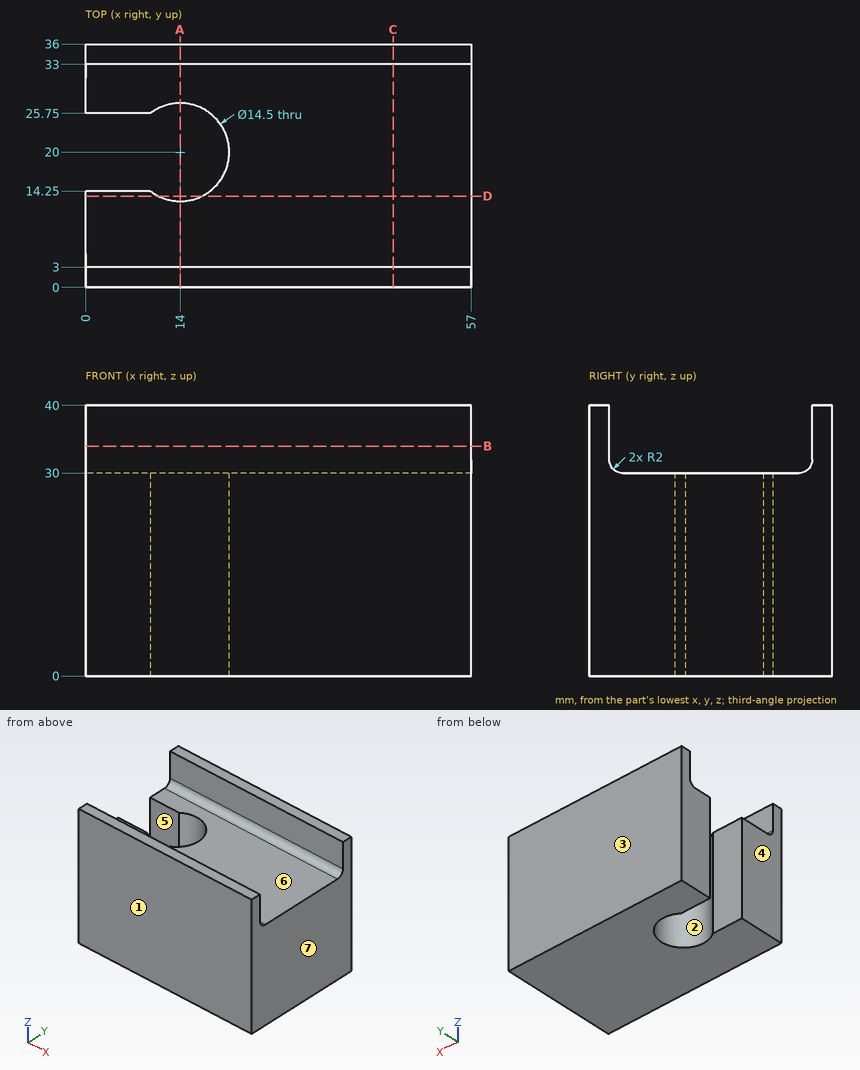
Verification items for this drawing (mm, ordinates from the low corner). A direction names the side the tool comes from. Round coordinates to 2 decimals unless told otherwise and drop trailing zeros. Order: outer loops, then holes, each group sorted by start corner. A loop starts at its lowest first (then second) coordinate and runs counter-clockwise, first axis right, second up.
1) Cross-section at D-D, the plane y = 13.5. Record the cut outline in (x, z), plus the area to 3 significant figures.
Geometry says:
outline: (0, 0) - (10.79, 0) - (10.79, 30) - (0, 30) - close; (17.21, 0) - (57, 0) - (57, 30) - (17.21, 30) - close
area: 1,520 mm2
2) Material ranges on line 1 (Y direction, x = 14, z = 22.75); line 2 (Y direction, x = 34, z = 38.5); line 3 (Z direction, x = 30, y = 16.5), recorded low to high.
Geometry says:
line 1: y = 0 to 12.75, 27.25 to 36
line 2: y = 0 to 3, 33 to 36
line 3: z = 0 to 30
3) Cross-section at B-B, the plane z = 34. Record the cut outline in (x, y).
Geometry says:
outline: (0, 0) - (57, 0) - (57, 3) - (0, 3) - close; (0, 33) - (57, 33) - (57, 36) - (0, 36) - close
4) Cross-section at A-A, the plane x = 14. Record the cut outline in (y, z).
Geometry says:
outline: (0, 0) - (12.75, 0) - (12.75, 30) - (5, 30) arc R2 cw to (3, 32) - (3, 40) - (0, 40) - close; (27.25, 0) - (36, 0) - (36, 40) - (33, 40) - (33, 32) arc R2 cw to (31, 30) - (27.25, 30) - close
5) Tool access check on the marked faces 5, 6 and 7. Record the directions out of +Z, -Z, +X, -X, +Y, -Y that give a thin tool (end or side, any length) a straight path to the whole face; none if there is none.
Geometry says:
face 5: +Z, -Z, -X
face 6: +Z, +X, -X
face 7: +Z, -Z, +X, +Y, -Y
6) Cross-section at C-C, the plane x = 45.5. Record the cut outline in (y, z), plus the area to 3 significant figures.
Geometry says:
outline: (0, 0) - (36, 0) - (36, 40) - (33, 40) - (33, 32) arc R2 cw to (31, 30) - (5, 30) arc R2 cw to (3, 32) - (3, 40) - (0, 40) - close
area: 1,140 mm2
7) Draft check along Y on the marked faces 1, 2, 3 and 4. Enter one of: +Y half, -Y half, draft (parallel to the pull), parting line (faces both ways), or undercut.
Geometry says:
face 1: -Y half
face 2: undercut
face 3: +Y half
face 4: draft
8) Depth check by flat-ended pin: pin 1 (2 mm diameter, centred on y = 11, z = 8.5, fed in from -X); pin 2 (13 mm diameter, centred on x = 20, y = 23, fed in from +Z). Enter the tip coordinate at first touch or a pass-through.
Geometry says:
pin 1: stops at x = 0
pin 2: stops at z = 30
